from build123d import *

# Parameters (mm, degrees)
PAD_DEPTH       = 45
SKETCH001_W     = 55
SKETCH001_H     = 10
PAD001_DEPTH    = 55
SKETCH002_R     = 3
POCKET_DEPTH    = 22
SKETCH003_R     = 2.5
POCKET001_DEPTH = 10
PAD002_DEPTH    = 60
SKETCH005_R     = 4
POCKET002_DEPTH = 22


with BuildPart() as part:
    # Sketch → Pad (new body)
    with BuildSketch(Plane.XY):
        with BuildLine():
            Line((0, 22), (42, 22))
            ThreePointArc((42, 0), (44.669271, 11), (42, 22))
            Line((42, 0), (0, 0))
            Line((0, 7), (0, 0))
            Line((38.9, 7), (0, 7))
            ThreePointArc((38.9, 7), (41.228437, 11), (38.9, 15))
            Line((0, 15), (38.9, 15))
            Line((0, 22), (0, 15))
        make_face()
    extrude(amount=PAD_DEPTH)

    # Sketch001 (on Face4 of Pad) → Pad001 (join)
    with BuildSketch(Plane.XZ):
        with Locations((14.5, 40)):
            Rectangle(SKETCH001_W, SKETCH001_H)
    extrude(amount=PAD001_DEPTH)

    # Sketch002 (on Face8 of Pad001) → Pocket (cut)
    with BuildSketch(Plane.XZ):
        with Locations((28, 20)):
            Circle(SKETCH002_R)
    extrude(amount=-POCKET_DEPTH, mode=Mode.SUBTRACT)

    # Sketch003 (on Face12 of Pocket) → Pocket001 (cut)
    with BuildSketch(Plane.XY.offset(45)):
        with Locations((35.5, -9)):
            Circle(SKETCH003_R)
        with Locations((35.5, -46)):
            Circle(SKETCH003_R)
        with Locations((-5.5, -27.5)):
            Circle(SKETCH003_R)
    extrude(amount=-POCKET001_DEPTH, mode=Mode.SUBTRACT)

    # Sketch004 (on Face5 of Pocket001) → Pad002 (join)
    with BuildSketch(Plane.XY.offset(45)):
        with BuildLine():
            Line((0, 22), (42, 22))
            Line((42, 22), (42, 0))
            Line((42, 0), (0, 0))
            Line((0, 0), (0, 7))
            Line((0, 7), (39, 7))
            ThreePointArc((39, 7), (41.232207, 11), (39, 15))
            Line((39, 15), (0, 15))
            Line((0, 15), (0, 22))
        make_face()
    extrude(amount=PAD002_DEPTH)

    # Sketch005 (on Face6 of Pad002) → Pocket002 (cut)
    with BuildSketch(Plane(origin=(0, 22, 0), x_dir=(-1, 0, 0), z_dir=(0, 1, 0))):
        with Locations((-30, 55)):
            Circle(SKETCH005_R)
        with Locations((-30, 75)):
            Circle(SKETCH005_R)
        with Locations((-30, 95)):
            Circle(SKETCH005_R)
    extrude(amount=-POCKET002_DEPTH, mode=Mode.SUBTRACT)


solid = part.part
Could you check a few things on this model? Use its own coordinates, in mm. A direction names the side the tool comes from. Coordinates: 2 decimals unless noted, no trailing zeros. Order: outer loops, then holes, each group sorted by start corner. A loop starts at its lowest first (then second) coordinate and runs counter-clockwise, first axis right, second up. Notation, with made-up numbers: (38, -4.5) -> (72, -4.5) arc R22 ccw to (72, 30.5) -> close; hole circle Ø11 at (8.5, 11). An arc over 180 degrees is marked (long way). One line per question, with ' | ' between items.
Q1. Imagine slicing it at C-C on y = -27.5. Please give me the cut outline in (x, z), and give its area (3 significant figures).
Return value:
outline: (-13, 35) -> (-8, 35) -> (-8, 45) -> (-13, 45) -> close; (-3, 35) -> (42, 35) -> (42, 45) -> (-3, 45) -> close | area: 500 mm²
Q2. Imagine slicing it at B-B on z = 75. Please give me the cut outline in (x, y), and give its area (3 significant figures).
Return value:
outline: (0, 0) -> (26, 0) -> (26, 7) -> (0, 7) -> close; (0, 15) -> (26, 15) -> (26, 22) -> (0, 22) -> close; (34, 0) -> (42, 0) -> (42, 22) -> (34, 22) -> (34, 15) -> (39, 15) arc R4.7 cw to (39, 7) -> (34, 7) -> close | area: 487 mm²
Q3. Imagine slicing it at A-A on x = 35.5. Please give me the cut outline in (y, z), and give its area (3 significant figures).
Return value:
outline: (-55, 35) -> (-48.5, 35) -> (-48.5, 45) -> (-55, 45) -> close; (-43.5, 35) -> (-11.5, 35) -> (-11.5, 45) -> (-43.5, 45) -> close; (-6.5, 35) -> (0, 35) -> (0, 0) -> (7, 0) -> (7, 105) -> (0, 105) -> (0, 45) -> (-6.5, 45) -> close; (15, 0) -> (22, 0) -> (22, 105) -> (15, 105) -> close | area: 1,920 mm²
Q4. I'm going to push flat-ended pins straight in: P1, Ø1.3, axis at x = 43, y = 9, coming from the +Z side; P2, Ø16.5, axis at x = 17.5, y = -35.5, coming from the -Z side; P3, Ø2, axis at x = 13, z = 28, coming from the -Y side. Where does each tip first touch, or does it pass through?
Return value:
P1: z = 45 | P2: z = 35 | P3: y = 0
Q5. If I drill on L1, parallel to Y at x = 24.5, z = 85.5; L2, parallel to Z at x = 28, y = 1; L3, parallel to Z at x = 30, y = 17, over which ranges is the centre line in solid material (lowest first)?
Return value:
L1: 0 to 7, 15 to 22 | L2: 0 to 17, 23 to 51.54, 58.46 to 71.54, 78.46 to 91.54, 98.46 to 105 | L3: 0 to 17.76, 22.24 to 51, 59 to 71, 79 to 91, 99 to 105
Q6. Thinking about a two-plate mould opening in X: for faces 4 (the face through (42, -27, 40)), 5 (the face through (30.867, 3.549, 71.095)), 6 (the face through (41.228, 10.932, 22.185)), which applies, pulls with the +X half, pulls with the -X half, needs draft (parallel to the pull), parting line crosses it, or undercut?
Return value:
face 4: pulls with the +X half | face 5: undercut | face 6: pulls with the -X half
Q7. On a 3-axis mill with a long thin cutter (end or side, diameter ignored), from which of +Z, -Z, +X, -X, +Y, -Y can I reach the whole of each face in a straight line? I mean faces 1 (the face through (21, 0, 17)), 2 (the face through (19, 7, 52)), 3 (the face through (28.154, 3.549, 91.451)). Say none if no direction works.
Return value:
face 1: -Z, +X, -X, -Y | face 2: +Z, -Z, -X | face 3: +Y, -Y
Q8. Imagine slicing it at D-D on z = 39.5. Please give me the cut outline in (x, y).
Return value:
outline: (-13, -55) -> (42, -55) -> (42, 0) arc R24 ccw to (42, 22) -> (0, 22) -> (0, 15) -> (38.9, 15) arc R4.6 cw to (38.9, 7) -> (0, 7) -> (0, 0) -> (-13, 0) -> close; hole circle Ø5 at (-5.5, -27.5); hole circle Ø5 at (35.5, -46); hole circle Ø5 at (35.5, -9)
